```python
from build123d import *

# Parameters (mm, degrees)
SKETCH1_W           = 24.5
SKETCH1_H           = 10
BOSS_EXTRUDE1_DEPTH = 1
SKETCH2_W           = 6.1
SKETCH2_H           = 3
BOSS_EXTRUDE2_DEPTH = 3.25
SKETCH4_W           = 6.1
SKETCH4_H           = 1
BOSS_EXTRUDE3_DEPTH = 1
SKETCH3_R           = 3.25
CUT_EXTRUDE1_DEPTH  = 3
FILLET1_R           = 0.2


with BuildPart() as part:
    # Sketch1 → Boss-Extrude1 (new body)
    with BuildSketch(Plane(origin=(0, 0, 0), x_dir=(1, 0, 0), z_dir=(0, 1, 0))):
        with Locations((-12.25, 5)):
            Rectangle(SKETCH1_W, SKETCH1_H)
    extrude(amount=BOSS_EXTRUDE1_DEPTH)

    # Sketch2 → Boss-Extrude2 (add)
    with BuildSketch(Plane(origin=(0, 1, 0), x_dir=(1, 0, 0), z_dir=(0, 1, 0))):
        with Locations((-19.65, 0.5)):
            Rectangle(SKETCH2_W, SKETCH2_H)
    extrude(amount=BOSS_EXTRUDE2_DEPTH)

    # Sketch4 → Boss-Extrude3 (add)
    with BuildSketch(Plane(origin=(0, 1, 0), x_dir=(-1, 0, 0), z_dir=(0, -1, 0))):
        with Locations((19.65, -0.5)):
            Rectangle(SKETCH4_W, SKETCH4_H)
    extrude(amount=BOSS_EXTRUDE3_DEPTH)

    # Sketch3 → Cut-Extrude1 (cut)
    with BuildSketch(Plane.XY.offset(1)):
        with Locations((-19.65, 4.25)):
            Circle(SKETCH3_R)
    extrude(amount=-CUT_EXTRUDE1_DEPTH, mode=Mode.SUBTRACT)

    # Fillet1
    fillet1_edges = [part.edges().sort_by_distance(p)[0] for p in [
        (-16.6, 3.127502784, -0.5),
        (-22.7, 3.127502784, -0.5),
    ]]
    fillet(fillet1_edges, radius=FILLET1_R)


solid = part.part
```
Can you work these out from the model? Positions are in its coordinate system, mm. A direction names the side the tool comes from. Coordinates: 2 decimals unless noted, no trailing zeros. Order: outer loops, then holes, each group sorted by start corner. A loop starts at its lowest first (then second) coordinate and runs counter-clockwise, first axis right, second up.
1. For faces 1 (the face through (-21.9, 1.6, -2)), 2 (the face through (-8.4, 0.5, 0)), 3 (the face through (-23.6, 0.5, 0)), 4 (the face through (-19.7, 1, -0.5)), which set-ups out of +Z, -Z, +X, -X, +Y, -Y let a thin tool reach every point of the face, with its end or its side?
2. If we section it at C-C (x = -10): Please give me the cut outline in (y, z), then the cut area to 3 significant figures.
3. I need wall thicknesses on line 1 (Z direction, x = -15.75, y = 0.85); line 2 (Z direction, x = -22.5, y = 1.65); line 3 (Y direction, x = -14.25, z = -3.25). Which ranges of each line are inside material? Lowest first, please.
4. If we section it at B-B (z = -0.5): Please give me the cut outline in (x, y).
5. I'm going to push flat-ended pins straight in: pin 1 (0.5 mm diameter, centred on x = -17.5, y = 2, fed in from -Z); pin 2 (0.8 mm diameter, centred on x = -23.5, y = 0.5, fed in from +Z); pin 3 (1 mm diameter, centred on x = -13.5, z = -7, fed in from +Y). Where does each tip first touch, or does it pass through?
6. If we section it at D-D (z = -9): Please give me the cut outline in (x, y).
7. If we section it at A-A (y = 0.3): Please give me the cut outline in (x, z).
Entries:
1. face 1: -Z, +X, -X, +Y
1. face 2: +Z, +X, +Y, -Y
1. face 3: +Z, -X, +Y, -Y
1. face 4: +Z, -Z, +Y
2. outline: (0, -10) - (1, -10) - (1, 0) - (0, 0) - close
2. area: 10.0 mm2
3. line 1: z = -10 to 0
3. line 2: z = -2 to 1
3. line 3: y = 0 to 1
4. outline: (-24.5, 0) - (0, 0) - (0, 1) - (-16.6, 1) - (-16.6, 2.31) arc R0.2 ccw to (-16.97, 2.42) arc R3.25 cw to (-22.33, 2.42) arc R0.2 ccw to (-22.7, 2.31) - (-22.7, 1) - (-24.5, 1) - close
5. pin 1: stops at z = -2
5. pin 2: stops at z = 0
5. pin 3: stops at y = 1
6. outline: (-24.5, 0) - (0, 0) - (0, 1) - (-24.5, 1) - close
7. outline: (-24.5, -10) - (0, -10) - (0, 0) - (-16.6, 0) - (-16.6, 1) - (-22.7, 1) - (-22.7, 0) - (-24.5, 0) - close
